Part print with two shaded views. Sizes in mm from the minimum x, y, z corner. Coordinates: 2 decimals unless noted, no trailing zeros. Loops run counter-clockwise (first coordinate to the right, second up) from the corner with the lowest first, then second, coordinate; pieces in that order, holes last.
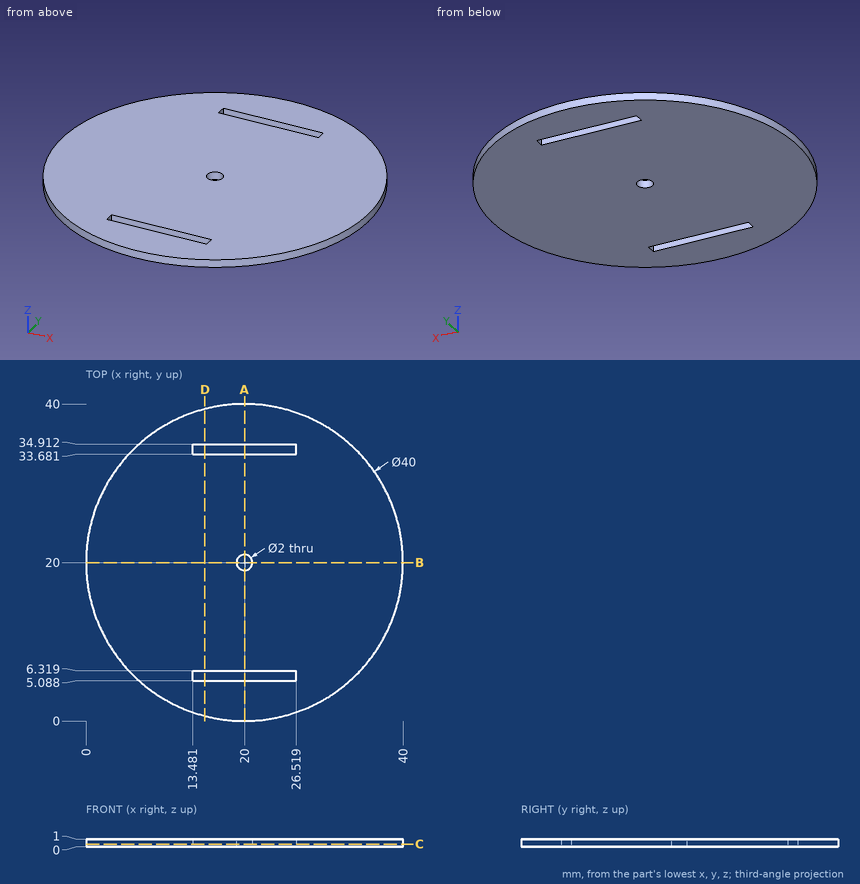
Q1. Drill centre lines: line 1 (Y direction, x = 20, z = 0.3); line 2 (Y direction, x = 23, z = 0.6); line 3 (Y direction, x = 18.5, z = 0.15). Where is each one in solid material? Low to high.
Answers:
line 1: y = 0 to 5.09, 6.32 to 19, 21 to 33.68, 34.91 to 40
line 2: y = 0.23 to 5.09, 6.32 to 33.68, 34.91 to 39.77
line 3: y = 0.06 to 5.09, 6.32 to 33.68, 34.91 to 39.94
Q2. Slice it at A-A (x = 20). List the corners of the cut face in (y, z).
Answers:
outline: (0, 0) - (5.09, 0) - (5.09, 1) - (0, 1) - close; (6.32, 0) - (19, 0) - (19, 1) - (6.32, 1) - close; (21, 0) - (33.68, 0) - (33.68, 1) - (21, 1) - close; (34.91, 0) - (40, 0) - (40, 1) - (34.91, 1) - close
Q3. Slice it at B-B (y = 20). List the corners of the cut face in (x, z).
Answers:
outline: (0, 0) - (19, 0) - (19, 1) - (0, 1) - close; (21, 0) - (40, 0) - (40, 1) - (21, 1) - close
Q4. Slice it at C-C (z = 0.35). List the corners of the cut face in (x, y), and give its area (3 significant figures).
Answers:
outline: circle Ø40 at (20, 20); hole (13.48, 5.09) - (26.52, 5.09) - (26.52, 6.32) - (13.48, 6.32) - close; hole (13.48, 33.68) - (26.52, 33.68) - (26.52, 34.91) - (13.48, 34.91) - close; hole circle Ø2 at (20, 20)
area: 1,220 mm2
Q5. Flat gauge pins, fed straight in: P1, Ø0.5, axis at y = 6, z = 0.5, coming from the +X side; P2, Ø1.8, axis at x = 20, y = 20, coming from the +Z side. Where does each tip first touch, or does it go through?
Answers:
P1: stops at x = 34.52
P2: passes through
Q6. Slice it at D-D (x = 15). List the corners of the cut face in (y, z) (1 decimal).
Answers:
outline: (0.6, 0) - (5.1, 0) - (5.1, 1) - (0.6, 1) - close; (6.3, 0) - (33.7, 0) - (33.7, 1) - (6.3, 1) - close; (34.9, 0) - (39.4, 0) - (39.4, 1) - (34.9, 1) - close
